from build123d import *

# Parameters (mm, degrees)
ESBO_O2_W                = 100
ESBO_O2_H                = 100
RESSALTO_EXTRUS_O1_DEPTH = 12.7
CORTE_EXTRUS_O1_DEPTH    = 72.842118566
ESBO_O7_R                = 2.95
CORTE_EXTRUS_O3_DEPTH    = 3.5
RESSALTO_EXTRUS_O4_DEPTH = 3.5
PADR_OCIRCULAR1_COUNT    = 26
FILETE2_R                = 5
FURO_ROSCADO_DE_M61_D    = 5


with BuildPart() as part:
    # Esboço2 → Ressalto-extrusão1 (new body)
    with BuildSketch(Plane(origin=(0, 0, 0), x_dir=(1, 0, 0), z_dir=(0, 1, 0))):
        Rectangle(ESBO_O2_W, ESBO_O2_H)
    extrude(amount=RESSALTO_EXTRUS_O1_DEPTH)

    # Esboço4 → Corte-extrusão1 (cut, through all)
    with BuildSketch(Plane(origin=(0, 0, 0), x_dir=(0, 0, -1), z_dir=(1, 0, 0))):
        Polygon((-30, 12.7), (-10, 12.7), (-7.75, 8.7), (-32.25, 8.7), align=None)
    corte_extrus_o1 = extrude(amount=-CORTE_EXTRUS_O1_DEPTH, mode=Mode.SUBTRACT)

    # Espelhar1: Corte-extrusão1 across plane
    add(corte_extrus_o1.mirror(Plane.XY), mode=Mode.SUBTRACT)

    # Esboço7 → Corte-extrusão3 (cut)
    with BuildSketch(Plane.XZ):
        with Locations(Location((0, 0, 0), (0, 0, 270))):
            Circle(ESBO_O7_R)
    extrude(amount=-CORTE_EXTRUS_O3_DEPTH, mode=Mode.SUBTRACT)

    # Esboço8 → Ressalto-extrusão4 (add)
    with BuildSketch(Plane(origin=(0, 0, 0), x_dir=(-1, 0, 0), z_dir=(0, -1, 0))):
        Polygon((0, -2.78), (-0.337974861, -2.93057554), (-0.337974861, -2.981739448), (0.337974861, -2.981739448), (0.337974861, -2.93057554), align=None)
    ressalto_extrus_o4 = extrude(amount=-RESSALTO_EXTRUS_O4_DEPTH)

    # PadrãoCircular1: Ressalto-extrusão4 ×26 about axis
    padr_ocircular1_axis = Axis((0, 0, 0), (0, 1, 0))
    for i in range(1, PADR_OCIRCULAR1_COUNT):
        add(ressalto_extrus_o4.rotate(padr_ocircular1_axis, i * 360 / PADR_OCIRCULAR1_COUNT))

    # Filete2
    filete2_edges = [part.edges().sort_by_distance(p)[0] for p in [
        (-50, 6.35, -50),
        (50, 6.35, -50),
        (50, 6.35, 50),
        (-50, 6.35, 50),
    ]]
    fillet(filete2_edges, radius=FILETE2_R)

    # Furo roscado de M61 (through all)
    with Locations(Plane(origin=(0, 0, 0), x_dir=(-1, 0, 0), z_dir=(0, -1, 0))):
        with Locations((-13.9125, -20), (-13.9125, 20)):
            Hole(FURO_ROSCADO_DE_M61_D / 2)


solid = part.part
Could you check a few things on this model? Use its own coordinates, in mm. A direction names the side the tool comes from. Round coordinates to 2 decimals unless told otherwise and drop trailing zeros. Write each loop counter-clockwise with the first axis right and the second up, starting at its lowest first coordinate (ties: lowest second). Pieces come first, ordered by that corner, then holes. Notation, with made-up numbers: (66.5, -26) - (108.5, -26) arc R8 ccw to (108.5, -20) - close; hole circle Ø10 at (70.5, 3). An arc over 180 degrees is marked (long way). Put each result on its own line as item: value. Start each with the question number.
(1) I want a section at B-B, the plane y = 10.25. Please give me the cut outline in (x, z), plus the area to 3 significant figures.
(2) Thinking about a two-plate mould opening in Z: for faces 1 (the flat face through (0, 11, 20)), 2 (the cylindrical face through (48, 6, 49)), 3 (the flat face through (-50, 5, 1)), which applies, released by +Z, released by -Z, zero draft, split by the parting line, or undercut?
(3) For faces 4 (the cylindrical face through (13.59, 6.44, -22.48)), 5 (the flat face through (0, 3.5, 0)), 6 (the flat face through (-25, 8.7, -20)), which set-ups out of +Z, -Z, +X, -X, +Y, -Y let a thin tool reach every point of the face, with its end or its side?
(4) Will these pins go through, and if not, where does the flat tip stop? pin 1 (3 mm diameter, centred on x = 13.91, z = -20, fed in from +Y); pin 2 (3 mm diameter, centred on x = -0.5, z = -0.5, fed in from -Y); pin 3 (4.5 mm diameter, centred on y = 11, z = -21, fed in from -X).
(5) I want a section at A-A, the plane z = 20. Please give me the cut outline in (x, y), plus the area to 3 significant figures.
(6) I need wall thicknesses on probe 1 along X at (y, z) = (5.75, 20); probe 2 along Z at (x, y) = (-4.5, 10); probe 3 along Y at (x, z) = (-21.5, 12). Which ranges of each line are inside material? Lowest first, please.
Here are the results:
1. outline: (-50, -45) arc R5 ccw to (-45, -50) - (45, -50) arc R5 ccw to (50, -45) - (50, 45) arc R5 ccw to (45, 50) - (-45, 50) arc R5 ccw to (-50, 45) - (-50, 31.38) - (0, 31.38) - (0, 8.62) - (-50, 8.62) - (-50, -8.62) - (0, -8.62) - (0, -31.38) - (-50, -31.38) - close; hole circle Ø5 at (13.91, -20); hole circle Ø5 at (13.91, 20)
1. area: 7,660 mm^2
2. face 1: undercut
2. face 2: released by +Z
2. face 3: zero draft
3. face 4: +Y, -Y
3. face 5: -Y
3. face 6: -X
4. pin 1: passes through
4. pin 2: stops at y = 3.5
4. pin 3: stops at x = 0
5. outline: (-50, 0) - (11.41, 0) - (11.41, 12.7) - (0, 12.7) - (0, 8.7) - (-50, 8.7) - close; (16.41, 0) - (50, 0) - (50, 12.7) - (16.41, 12.7) - close
5. area: 1,010 mm^2
6. probe 1: x = -50 to 11.41, 16.41 to 50
6. probe 2: z = -50 to -31.52, -8.48 to 8.48, 31.52 to 50
6. probe 3: y = 0 to 8.7
